Input: part model. Units: mm. Frame: model coordinates. Face numbers are marked on the shaded views. A direction names the side the tool comes from. Round coordinates to 2 decimals unless told otherwise and drop trailing zeros. Order: outer loops, then holes, each group sorted by start corner. A loop starts at its lowest first (then second) coordinate and runs counter-clockwise, first axis right, second up. Notation, with made-up numbers: (-5.5, 46.25) -> (13.5, 46.25) arc R27 cw to (13.5, 67.25) -> close; hole circle Ø3 at (59, 13.5). An arc over 180 degrees is marked (long way). Use a Markdown table: item, result.
from build123d import *

# Parameters (mm, degrees)
F0_R     = 3.81
F1_DEPTH = 0.889
F2_R     = 1.27
F3_DEPTH = 3.81
F5_DEPTH = 0.8636


with BuildPart() as f1:
    # F0 (on Top) → F1 (new body)
    with BuildSketch(Plane.XY):
        Circle(F0_R)
    extrude(amount=F1_DEPTH)

    # F2 (on face) → F3 (join)
    with BuildSketch(Plane.XY.offset(0.889)):
        Circle(F2_R)
    extrude(amount=F3_DEPTH)

    # F4 (on face) → F5 (cut)
    with BuildSketch(Plane(origin=(0, 0, 0), x_dir=(1, 0, 0), z_dir=(0, 0, -1))):
        Polygon((2.963077, 0.36432), (1.166028, 2.74826), (-1.797049, 2.38394), (-2.963077, -0.36432), (-1.166028, -2.74826), (1.797049, -2.38394), align=None)
    extrude(amount=-F5_DEPTH, mode=Mode.SUBTRACT)


solid = f1.part
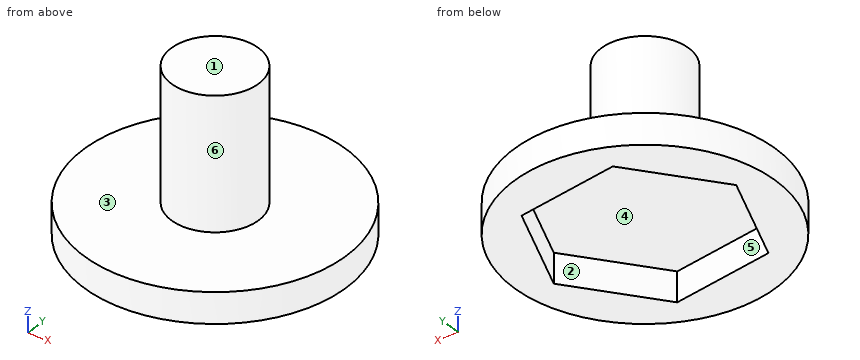
1) Set-up query: the marked faces 1 and 2. Return all of +Z, -Z, +X, -X, +Y, -Y with unobstructed straight access to the full face (end or side cutting, diameter ignored); none if empty.
Results found:
| item | result |
|---|---|
| face 1 | +Z, +X, -X, +Y, -Y |
| face 2 | -Z |
2) Cut plane D-D on y = 1. Return loops of the section in (x, z), and give its area (3 significant figures).
Results found:
| item | result |
|---|---|
| outline | (-3.68, 0) -> (-2.48, 0) -> (-2.48, 0.86) -> (2.38, 0.86) -> (2.38, 0) -> (3.68, 0) -> (3.68, 0.89) -> (0.78, 0.89) -> (0.78, 4.7) -> (-0.78, 4.7) -> (-0.78, 0.89) -> (-3.68, 0.89) -> close |
| area | 8.30 mm² |
3) Pull-direction query (Y, two-part tool) for the marked faces 3, 4, 5 and 6; classes: +Y half, -Y half, draft (parallel to the pull), parting line (faces both ways), or undercut.
Results found:
| item | result |
|---|---|
| face 3 | draft |
| face 4 | undercut |
| face 5 | undercut |
| face 6 | parting line |
4) Line query: L1, parallel to Z at x = -1.75, y = 2.75; L2, parallel to Z at x = 0.25, y = 0.25; L3, parallel to X at y = -0.25, z = 1.2. Output: solid intervals per line, ascending. Write a range as [from, to].
Results found:
| item | result |
|---|---|
| L1 | z = [0, 0.89] |
| L2 | z = [0.86, 4.7] |
| L3 | x = [-1.25, 1.25] |
5) Cut plane B-B on y = 2. Return loops of the section in (x, z).
Results found:
| item | result |
|---|---|
| outline | (-3.24, 0) -> (-1.73, 0) -> (-1.73, 0.86) -> (1.96, 0.86) -> (1.96, 0) -> (3.24, 0) -> (3.24, 0.89) -> (-3.24, 0.89) -> close |
6) Cut plane C-C on z = 1.3. Return loops of the section in (x, y).
Results found:
| item | result |
|---|---|
| outline | circle Ø2.54 at (0, 0) |
7) Cut plane A-A on x = 1.5. Return loops of the section in (y, z), and give its area (3 significant figures).
Results found:
| item | result |
|---|---|
| outline | (-3.5, 0) -> (-2.31, 0) -> (-2.31, 0.86) -> (2.42, 0.86) -> (2.42, 0) -> (3.5, 0) -> (3.5, 0.89) -> (-3.5, 0.89) -> close |
| area | 2.15 mm² |
8) Pin query (flat end, axial travel): pin 1 Ø2 at (x, z) = (2.5, 1.5) entering from +Y; pin 2 Ø1 at (x, y) = (-1.5, -2.5) entering from +Z; pin 3 Ø4.5 at (x, y) = (0, -1) entering from -Z; pin 4 Ø1 at (x, z) = (1.5, 3) entering from +Y. Return the tip coordinate at first contact, or that it passes through.
Results found:
| item | result |
|---|---|
| pin 1 | stops at y = 3.41 |
| pin 2 | stops at z = 0.89 |
| pin 3 | stops at z = 0 |
| pin 4 | stops at y = 0.78 |
